Build history of the part. All positions in model axes, mm. Face numbers are marked on the shaded views. A direction names the side the tool comes from. Give positions to 0.01 mm unless a question says otherwise; leave off trailing zeros. Write each loop counter-clockwise with the first axis right and the second up, starting at its lowest first coordinate (ties: lowest second). Pieces come first, ordered by that corner, then holes. Notation, with made-up numbers: (-20.5, 6.5) -> (-15.5, 6.5) arc R10 ccw to (-15.5, 12.5) -> close; hole circle Ø8 at (-33, 47). An arc over 180 degrees is marked (long way). One line per question, with ' | ' between items. Start each with the question number.
(1) Band-saw the part on C-C, the plane z = 8. Give the cut face in (x, y), and give its area (3 significant figures).
(2) Band-saw the part on A-A, the plane y = 6. Give the cut face in (x, z), and give its area (3 significant figures).
(3) Pin check, flat tips, straight feed: P1, Ø3, axis at y = -12, z = 21, coming from the -X side; P2, Ø3.5, axis at y = -16, z = 36, coming from the +X side; P3, Ø10.5, axis at x = -31, y = 6, coming from the +Z side; P4, Ø5, axis at y = 15, z = 35, coming from the -X side. Stop position of each tip, or through.
(4) Pull direction Y, two halves, no side cores. Call the marked faces 1, 2 and 3: released by +Y, released by -Y, zero draft, split by the parting line, or undercut.
(5) Tool access for the marked faces 4, 5 and 6: list every direction of +Z, -Z, +X, -X, +Y, -Y with a clear straight run to the whole face (end or side of a thin tool).
(6) Drill centre lines: probe 1 along Z at (x, y) = (-1.3, -16); probe 2 along Z at (x, y) = (-32, 12); probe 3 along X at (y, z) = (-17.5, 34). Where is each one in solid material? Low to high. Write a range as from..to.
(7) Band-saw the part on D-D, the plane z = 20. Give the cut face in (x, y), and give its area (3 significant figures).
(8) Band-saw the part on B-B, the plane x = -10. Give the cut face in (y, z), and give its area (3 significant figures).
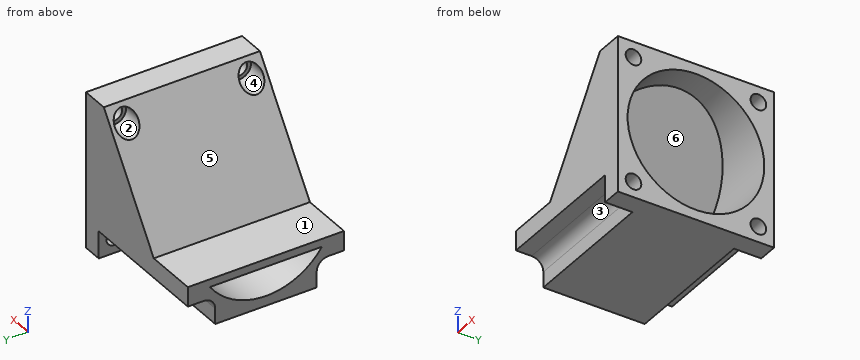
from build123d import *

# Parameters (mm, degrees)
PAD_DEPTH       = 20
SKETCH001_R     = 17.5
POCKET_DEPTH    = 40.001
PAD001_DEPTH    = 20
SKETCH003_R     = 3
POCKET001_DEPTH = 35
SKETCH004_R     = 2
POCKET002_DEPTH = 40.001


with BuildPart() as part:
    # Sketch → Pad (new body, symmetric)
    with BuildSketch(Plane.XZ):
        Polygon((-40, 0), (0, 0), (0, 40), (-5, 40), (-26.006226, 10), (-40, 10), align=None)
    extrude(amount=PAD_DEPTH, both=True)

    # Sketch001 → Pocket (cut, through all)
    with BuildSketch(Plane.YZ):
        with Locations((0, 20)):
            Circle(SKETCH001_R)
    extrude(amount=-POCKET_DEPTH, mode=Mode.SUBTRACT)

    # Sketch002 → Pad001 (join, symmetric)
    with BuildSketch(Plane.XZ):
        Polygon((-5, 40), (-7, 40), (-26.605811, 12), (-40, 12), (-40, 10), (-26.006226, 10), align=None)
    extrude(amount=PAD001_DEPTH, both=True)

    # Sketch003 (on Face6 of Pad001) → Pocket001 (cut)
    with BuildSketch(Plane(origin=(-40, 0, 0), x_dir=(0, 0, -1), z_dir=(-1, 0, 0))):
        with Locations((-36, 16)):
            Circle(SKETCH003_R)
        with BuildLine():
            Line((-4, 13), (4.613364, 13))
            Line((4.613364, 13), (4.613364, 24.650373))
            Line((4.613364, 24.650373), (-7, 24.650373))
            Line((-7, 24.650373), (-7, 16))
            ThreePointArc((-7, 16), (-6.12132, 13.87868), (-4, 13))
        make_face()
    pocket001 = extrude(amount=-POCKET001_DEPTH, mode=Mode.SUBTRACT)

    # Mirrored: Pocket001 across XZ
    add(pocket001.mirror(Plane.XZ), mode=Mode.SUBTRACT)

    # Sketch004 → Pocket002 (cut, through all)
    with BuildSketch(Plane.YZ):
        with Locations((16, 36)):
            Circle(SKETCH004_R)
        with Locations((16, 4)):
            Circle(SKETCH004_R)
        with Locations((-16, 4)):
            Circle(SKETCH004_R)
        with Locations((-16, 36)):
            Circle(SKETCH004_R)
    extrude(amount=-POCKET002_DEPTH, mode=Mode.SUBTRACT)


solid = part.part
Results:
1) outline: (-40, -20) -> (0, -20) -> (0, -12.74) -> (-40, -12.74) -> close; (-40, 12.74) -> (0, 12.74) -> (0, 20) -> (-40, 20) -> close | area: 581 mm²
2) outline: (-40, 0) -> (0, 0) -> (0, 3.56) -> (-40, 3.56) -> close; (-40, 10) -> (-26.01, 10) -> (-7.49, 36.44) -> (0, 36.44) -> (0, 40) -> (-7, 40) -> (-26.61, 12) -> (-40, 12) -> close | area: 250 mm²
3) P1: stops at x = -21.35 | P2: passes through | P3: stops at z = 13.22 | P4: stops at x = -12.25
4) face 1: zero draft | face 2: undercut | face 3: released by -Y
5) face 4: -X | face 5: +Z, -X, +Y, -Y | face 6: +X
6) probe 1: z = 0..2, 6..12.91, 27.09..34, 38..40 | probe 2: z = 0..7.26, 10..12 | probe 3: x = -5..0
7) outline: (-21, -20) -> (0, -20) -> (0, -17.5) -> (-19, -17.5) -> (-19, 17.5) -> (0, 17.5) -> (0, 20) -> (-21, 20) -> close | area: 175 mm²
8) outline: (-20, 7) -> (-16, 7) arc R3 cw to (-13, 4) -> (-13, 0) -> (13, 0) -> (13, 4) arc R3 cw to (16, 7) -> (20, 7) -> (20, 35.72) -> (18.99, 35.72) arc R3 cw to (13.01, 35.72) -> (-13.01, 35.72) arc R3 cw to (-18.99, 35.72) -> (-20, 35.72) -> close; hole (-11.87, 32.86) arc R17.5 ccw (long way) to (11.87, 32.86) -> close | area: 423 mm²
